Verification items for the finished model (mm, model axes). A direction names the side the tool comes from. Round coordinates to 2 decimals unless told otherwise and drop trailing zeros. Loops run counter-clockwise (first coordinate to the right, second up) from the corner with the lowest first, then second, coordinate; pieces in that order, holes last. Notation, with made-up numbers: (29, -9.75) -> (74, -9.75) arc R14 ccw to (74, -2.75) -> close; hole circle Ø7 at (31, -12.75). An arc over 180 degrees is marked (long way). Write item = value, one per line. Start each with the question number.
```python
from build123d import *

# Parameters (mm, degrees)
SKETCH1_W                    = 1648
SKETCH1_H                    = 125
BASE_FLANGE1_DEPTH           = 4
EDGE_FLANGE1_STRIP_W         = 28
EDGE_FLANGE1_STRIP_H         = 4
EDGE_FLANGE1_STRIP_CUT_DEPTH = 1648
EDGE_FLANGE1_DEPTH           = 1648
EDGE_FLANGE2_STRIP_W         = 28
EDGE_FLANGE2_STRIP_H         = 4
EDGE_FLANGE2_STRIP_CUT_DEPTH = 1648
EDGE_FLANGE2_DEPTH           = 1648


# Sheet-metal steps are written as plain solids
with BuildPart() as part:
    # Sketch1 → Base-Flange1 (new body)
    with BuildSketch(Plane.XY):
        with Locations((-340.8723099, 44.386657102)):
            Rectangle(SKETCH1_W, SKETCH1_H)
    extrude(amount=-BASE_FLANGE1_DEPTH)

    # Edge-Flange1 strip (across the edge) → Edge-Flange1 strip cut (cut)
    with BuildSketch(Plane(origin=(483.1276901, 106.886657102, 0), x_dir=(0, -1, 0), z_dir=(-1, 0, 0))):
        with Locations((-4, -2)):
            Rectangle(EDGE_FLANGE1_STRIP_W, EDGE_FLANGE1_STRIP_H)
    extrude(amount=EDGE_FLANGE1_STRIP_CUT_DEPTH, mode=Mode.SUBTRACT)

    # Edge-Flange1 section (across the edge) → Edge-Flange1 (add)
    with BuildSketch(Plane(origin=(483.1276901, 106.886657102, 0), x_dir=(0, -1, 0), z_dir=(-1, 0, 0))):
        with BuildLine():
            Line((0, 6), (0, 58))
            Line((0, 58), (4, 58))
            Line((4, 58), (4, 6))
            ThreePointArc((4, 6), (5.757359313, 1.757359313), (10, 0))
            Line((10, 0), (10, -4))
            ThreePointArc((10, -4), (2.928932188, -1.071067812), (0, 6))
        make_face()
    extrude(amount=EDGE_FLANGE1_DEPTH)

    # Edge-Flange2 strip (across the edge) → Edge-Flange2 strip cut (cut)
    with BuildSketch(Plane(origin=(-1164.8723099, -18.113342898, 0), x_dir=(0, 1, 0), z_dir=(1, 0, 0))):
        with Locations((-4, -2)):
            Rectangle(EDGE_FLANGE2_STRIP_W, EDGE_FLANGE2_STRIP_H)
    extrude(amount=EDGE_FLANGE2_STRIP_CUT_DEPTH, mode=Mode.SUBTRACT)

    # Edge-Flange2 section (across the edge) → Edge-Flange2 (add)
    with BuildSketch(Plane(origin=(-1164.8723099, -18.113342898, 0), x_dir=(0, 1, 0), z_dir=(1, 0, 0))):
        with BuildLine():
            Line((0, 6), (0, 58))
            Line((0, 58), (4, 58))
            Line((4, 58), (4, 6))
            ThreePointArc((4, 6), (5.757359313, 1.757359313), (10, 0))
            Line((10, 0), (10, -4))
            ThreePointArc((10, -4), (2.928932188, -1.071067812), (0, 6))
        make_face()
    extrude(amount=EDGE_FLANGE2_DEPTH)


solid = part.part
```
(1) Access from +Z, -Z, +X, -X, +Y, -Y to the whole of each face (thin tool, end or side, straight path). Record for faces 4 (the flat face through (-352, -14.113, 32)), 5 (the flat face through (-352, -18.113, 32)).
(2) Draft check along Y on faces 1 (the flat face through (-329, 102.887, 32)), 2 (the flat face through (-329, 106.887, 32)), 3 (the flat face through (483.128, 44.7, -0.4)). Enter one of: +Y half, -Y half, draft (parallel to the pull), parting line (faces both ways), or undercut.
(3) Section check B-B on x = -956. Enter the section's corners in (y, z), then the cut area to 3 significant figures.
(4) Depth check by flat-ended pin: pin 1 Ø10 at (x, y) = (77.5, 72.5) entering from +Z. Enter the tip coordinate at first touch or a pass-through.
(5) Section check A-A on z = 17.5. Enter the section's corners in (x, y).
(6) Scan lines: line 1 (Y direction, x = -150, z = 34); line 2 (Z direction, x = 392, y = 9.5); line 3 (Y direction, x = -955, z = -1). Record each from-to range of solid material in increasing order. Write a range as [from, to].
(7) Section check C-C on y = 42.5. Enter the section's corners in (x, z).
Computed values:
q1.face_4 = +Z, +X, -X
q1.face_5 = +Z, -Z, +X, -X, -Y
q2.face_1 = undercut
q2.face_2 = +Y half
q2.face_3 = draft
q3.outline = (-18.11, 6) arc R10 ccw to (-8.11, -4) -> (96.89, -4) arc R10 ccw to (106.89, 6) -> (106.89, 58) -> (102.89, 58) -> (102.89, 6) arc R6 cw to (96.89, 0) -> (-8.11, 0) arc R6 cw to (-14.11, 6) -> (-14.11, 58) -> (-18.11, 58) -> close
q3.area = 937 mm²
q4.pin_1 = 0
q5.outline = (-1164.87, -18.11) -> (483.13, -18.11) -> (483.13, -14.11) -> (-1164.87, -14.11) -> close; (-1164.87, 102.89) -> (483.13, 102.89) -> (483.13, 106.89) -> (-1164.87, 106.89) -> close
q6.line_1 = [-18.11, -14.11], [102.89, 106.89]
q6.line_2 = [-4, 0]
q6.line_3 = [-15.25, 104.03]
q7.outline = (-1164.87, -4) -> (483.13, -4) -> (483.13, 0) -> (-1164.87, 0) -> close
